```python
from build123d import *

# Parameters (mm, degrees)
RESSALTO_EXTRUS_O1_DEPTH        = 8.5
ESBO_O8_W                       = 19
ESBO_O8_H                       = 1.5
CORTE_EXTRUS_O1_DEPTH           = 3
ESBO_O5_W                       = 19
ESBO_O5_H                       = 1.5
CORTE_EXTRUS_O2_DEPTH           = 3
ESBO_O11_R                      = 2.25
CORTE_EXTRUS_O6_DEPTH           = 9.5
ESBO_O12_R                      = 2.25
CORTE_EXTRUS_O7_DEPTH           = 9.5
ESBO_O15_R                      = 6.5
CORTE_EXTRUS_O12_DEPTH          = 4
RESSALTO_EXTRUS_O2_DEPTH        = 4
ESBO_O17_R                      = 1.8
ESBO_O17_R_2                    = 1.7
CORTE_EXTRUS_O13_DEPTH          = 1.6
ESBO_O8_4_W                     = 19
ESBO_O8_4_H                     = 1.5
CORTE_EXTRUS_O14_DEPTH          = 3
ESBO_O11_7_R                    = 1.7
CORTE_EXTRUS_O18_DEPTH          = 9.5
RESSALTO_EXTRUS_O3_DEPTH        = 70
SKIZZE1_W                       = 7.6
SKIZZE1_H                       = 2
AUFSATZ_LINEAR_AUSTRAGEN1_DEPTH = 15
SKETCH1_R                       = 1.75
CUT_EXTRUDE1_DEPTH              = 10


with BuildPart() as part:
    # Esboço4 → Ressalto-extrusão1 (new body)
    with BuildSketch(Plane.XY):
        Polygon((-80, 16.5), (30, 16.5), (30, 6.85), (-30, 6.85), (-30, -6.85), (30, -6.85), (30, -16.5), (-80, -16.5), align=None)
    extrude(amount=RESSALTO_EXTRUS_O1_DEPTH)

    # Esboço8 → Corte-extrusão1 (cut)
    with BuildSketch(Plane(origin=(-30, -6.85, 8.5), x_dir=(1, 0, 0), z_dir=(0, 1, 0))):
        with Locations((15.5, 7.75)):
            Rectangle(ESBO_O8_W, ESBO_O8_H)
    extrude(amount=-CORTE_EXTRUS_O1_DEPTH, mode=Mode.SUBTRACT)

    # Esboço5 → Corte-extrusão2 (cut)
    with BuildSketch(Plane(origin=(-30, 6.85, 8.5), x_dir=(1, 0, 0), z_dir=(0, 1, 0))):
        with Locations((15.5, 7.75)):
            Rectangle(ESBO_O5_W, ESBO_O5_H)
        with Locations((45.5, 7.75)):
            Rectangle(ESBO_O5_W, ESBO_O5_H)
    extrude(amount=CORTE_EXTRUS_O2_DEPTH, mode=Mode.SUBTRACT)

    # Esboço11 → Corte-extrusão6 (cut, through all)
    with BuildSketch(Plane.XY.offset(8.5)):
        with Locations((-65, 10)):
            Circle(ESBO_O11_R)
    extrude(amount=-CORTE_EXTRUS_O6_DEPTH, mode=Mode.SUBTRACT)

    # Esboço12 → Corte-extrusão7 (cut, through all)
    with BuildSketch(Plane(origin=(-80, 16.5, 8.5), x_dir=(-1, 0, 0), z_dir=(0, 0, -1))):
        with Locations((-15, -19.5)):
            Circle(ESBO_O12_R)
    extrude(amount=CORTE_EXTRUS_O7_DEPTH, mode=Mode.SUBTRACT)

    # Esboço15 → Corte-extrusão12 (cut)
    with BuildSketch(Plane(origin=(-30, -6.85, 0), x_dir=(0, 0, 1), z_dir=(-1, 0, 0))):
        with Locations((0, 6.85)):
            Circle(ESBO_O15_R)
    extrude(amount=CORTE_EXTRUS_O12_DEPTH, mode=Mode.SUBTRACT)

    # Esboço16 → Ressalto-extrusão2 (add)
    with BuildSketch(Plane(origin=(-34, -6.5, 0), x_dir=(0, 0, -1), z_dir=(1, 0, 0))):
        with BuildLine():
            Line((0, 2), (0, 11))
            ThreePointArc((0, 11), (-4.5, 6.5), (0, 2))
        make_face()
    extrude(amount=RESSALTO_EXTRUS_O2_DEPTH)

    # Esboço17 → Corte-extrusão13 (cut)
    with BuildSketch(Plane(origin=(-80, 16.5, 0), x_dir=(-1, 0, 0), z_dir=(0, 0, -1))):
        with Locations((-5, -3)):
            Circle(ESBO_O17_R)
        with Locations((-5, -26)):
            Circle(ESBO_O17_R)
        with Locations((-52, -26)):
            Circle(ESBO_O17_R)
        with Locations((-52, -3)):
            Circle(ESBO_O17_R)
        with Locations((-107, -26)):
            Circle(ESBO_O17_R_2)
        with Locations((-107, -3)):
            Circle(ESBO_O17_R)
    extrude(amount=-CORTE_EXTRUS_O13_DEPTH, mode=Mode.SUBTRACT)

    # Esboço8<4> → Corte-extrusão14 (cut)
    with BuildSketch(Plane(origin=(-30, -6.85, 8.5), x_dir=(1, 0, 0), z_dir=(0, 1, 0))):
        with Locations((15.5, 7.75)):
            Rectangle(ESBO_O8_4_W, ESBO_O8_4_H)
        with Locations((45.5, 7.75)):
            Rectangle(ESBO_O8_4_W, ESBO_O8_4_H)
    extrude(amount=-CORTE_EXTRUS_O14_DEPTH, mode=Mode.SUBTRACT)

    # Esboço11<7> → Corte-extrusão18 (cut, through all)
    with BuildSketch(Plane.XY.offset(8.5)):
        with Locations((0, -11.5)):
            Circle(ESBO_O11_7_R)
        with Locations((0, 11.6)):
            Circle(ESBO_O11_7_R)
    extrude(amount=-CORTE_EXTRUS_O18_DEPTH, mode=Mode.SUBTRACT)

    # Esboço18 → Ressalto-extrusão3 (add)
    with BuildSketch(Plane(origin=(-30, -4.5, 0), x_dir=(0, 0, 1), z_dir=(-1, 0, 0))):
        with BuildLine():
            Line((0, 2.5), (0, 6.5))
            ThreePointArc((0, 6.5), (2, 4.5), (0, 2.5))
        make_face()
    extrude(amount=-RESSALTO_EXTRUS_O3_DEPTH)

    # Skizze1 → Aufsatz-Linear austragen1 (add)
    with BuildSketch(Plane(origin=(0, -6.85, 0), x_dir=(1, 0, 0), z_dir=(0, 1, 0))):
        with Locations((26.2, -7.5)):
            Rectangle(SKIZZE1_W, SKIZZE1_H)
    extrude(amount=AUFSATZ_LINEAR_AUSTRAGEN1_DEPTH)

    # Sketch1 → Cut-Extrude1 (cut)
    with BuildSketch(Plane.XY.offset(8.5)):
        with Locations((20, 13)):
            Circle(SKETCH1_R)
        with Locations((20, -13)):
            Circle(SKETCH1_R)
    extrude(amount=-CUT_EXTRUDE1_DEPTH, mode=Mode.SUBTRACT)


solid = part.part
```
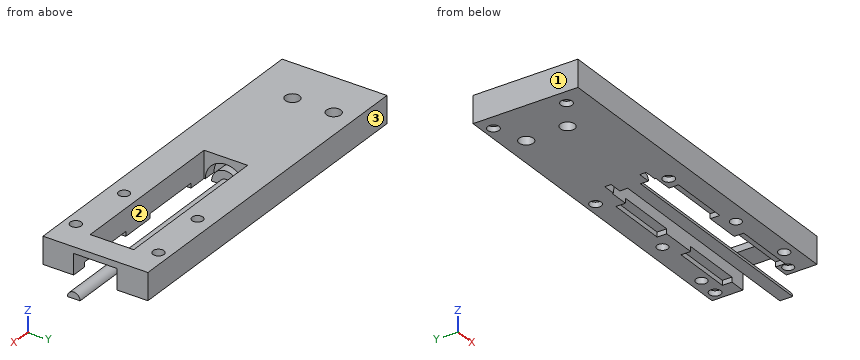
Can you work these out from the model? Positions are in its coordinate system, mm. Face numbers are marked on the shaded views. Give positions to 0.01 mm unless a question says otherwise; leave off trailing zeros. Order: outer loops, then holes, each group sorted by start corner. A loop starts at its lowest first (then second) coordinate and runs counter-clockwise, first axis right, second up. Notation, with made-up numbers: M 6,50 L 48,50 A27 ccw 48,77 Z; hole C 5.5,24.5 d5. An arc over 180 degrees is marked long. One line per item, written item: value.
1) Please list where these lines run through material, in increasing order: line 1 along Y through (x, z) = (-75, 1); line 2 along Y through (x, z) = (-65, 2.75); line 3 along Y through (x, z) = (0, 6).
Answer sheet:
line 1: y = -16.5 to -11.3, -7.7 to 11.7, 15.3 to 16.5
line 2: y = -16.5 to -5.25, -0.75 to 7.75, 12.25 to 16.5
line 3: y = -16.5 to -13.2, -9.8 to -6.85, 6.85 to 9.9, 13.3 to 16.5
2) I want a section at B-B, the plane x = 27. List the corners of the cut face in (y, z) for me.
Answer sheet:
outline: M -16.5,0 L -11.2,0 L -11.2,1.6 L -7.8,1.6 L -7.8,0 L -6.85,0 L -6.85,6.5 L 6.85,6.5 L 6.85,0 L 11.7,0 L 11.7,1.6 L 15.3,1.6 L 15.3,0 L 16.5,0 L 16.5,8.5 L -16.5,8.5 Z; M -2,0 L 2,0 A2 ccw Z
3) I want a section at D-D, the plane x = -28. List the corners of the cut face in (y, z) for me.
Answer sheet:
outline: M -16.5,0 L -11.3,0 L -11.3,1.6 L -7.7,1.6 L -7.7,0 L -6.85,0 L -6.85,8.5 L -16.5,8.5 Z; M -2,0 L 2,0 A2 ccw Z; M 6.85,0 L 11.7,0 L 11.7,1.6 L 15.3,1.6 L 15.3,0 L 16.5,0 L 16.5,8.5 L 6.85,8.5 Z
4) For P1, Ø2, axis at y = 2, z = 3, coming from the +X side; P2, Ø1.8, axis at x = -75, y = 13.5, coming from the -Z side, each with a flat end and sliding along its axis, tell me the tip position at first contact or that it passes through.
Answer sheet:
P1: stops at x = -30
P2: stops at z = 1.6
5) I want a section at C-C, the plane y = -3. List the corners of the cut face in (x, z) for me, plus the area to 3 significant figures.
Answer sheet:
outline: M -80,0 L -67.25,0 L -67.25,8.5 L -80,8.5 Z; M -62.75,0 L -30,0 L -30,3.35 L -34,3.35 L -34,5.77 L -30,5.77 L -30,8.5 L -62.75,8.5 Z; M 22.4,6.5 L 30,6.5 L 30,8.5 L 22.4,8.5 Z
area: 392 mm^2
6) We'd pull the mould along X, two halves only. Please class the marked faces 1, 2 and 3: released by +X, released by -X, zero draft, split by the parting line, or undercut.
Answer sheet:
face 1: released by -X
face 2: undercut
face 3: zero draft
7) I want a section at A-A, the plane x = 11. List the corners of the cut face in (y, z) for me, plus the area to 3 significant figures.
Answer sheet:
outline: M -16.5,0 L -9.85,0 L -9.85,1.5 L -6.85,1.5 L -6.85,8.5 L -16.5,8.5 Z; M -2,0 L 2,0 A2 ccw Z; M 6.85,1.5 L 9.85,1.5 L 9.85,0 L 16.5,0 L 16.5,8.5 L 6.85,8.5 Z
area: 161 mm^2
